```python
from build123d import *

# Parameters (mm, degrees)
F0_R     = 15
F1_DEPTH = 2.5
F2_R     = 5.5
F3_DEPTH = 5
F4_R     = 3
F5_DEPTH = 25
F6_SIZE  = 1


with BuildPart() as f1:
    # F0 (on Front) → F1 (new body)
    with BuildSketch(Plane.XZ):
        Circle(F0_R)
    extrude(amount=F1_DEPTH)

    # F2 (on face) → F3 (join)
    with BuildSketch(Plane.XZ.offset(2.5)):
        Circle(F2_R)
    extrude(amount=F3_DEPTH)

    # F4 (on face) → F5 (cut)
    with BuildSketch(Plane.XZ.offset(7.5)):
        Circle(F4_R)
    extrude(amount=-F5_DEPTH, mode=Mode.SUBTRACT)

    # F6
    f6_edges = [f1.edges().sort_by_distance(p)[0] for p in [
        (-5.5, -7.5, 0),
        (-15, 0, 0),
    ]]
    chamfer(f6_edges, length=F6_SIZE)


solid = f1.part
```
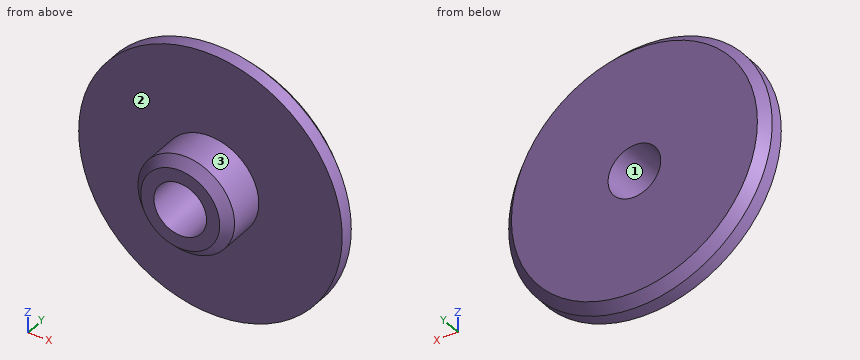
Here's how the part is built. I have some questions about the finished solid (model axes, mm). Face numbers are marked on the shaded views. Give positions to 0.01 mm unless a question says otherwise; leave off trailing zeros. Order: outer loops, then holes, each group sorted by start corner. A loop starts at its lowest first (then second) coordinate and runs counter-clockwise, first axis right, second up. Notation, with made-up numbers: M -3.5,-30 L 40.5,-30 A20 cw 40.5,9 Z; hole C 88,51 d3. An arc over 180 degrees is marked long. Use a Markdown table: item, result. Add a question column.
1. Suppose I cut it at B-B (z = 0). List the corners of the cut face in (x, y) for me, and give its area (3 significant figures).
2. Suppose I cut it at C-C (y = -1.5). List the corners of the cut face in (x, z) for me, and give its area (3 significant figures).
3. Suppose I cut it at A-A (x = 0). List the corners of the cut face in (y, z) for me, and give its area (3 significant figures).
4. Suppose I cut it at D-D (y = -3.5). List the corners of the cut face in (x, z) for me.
5. If we mould it in two halves opening along X, with no side actions, what happens to the marked faces 1, 2 and 3? For each: +X half, -X half, draft (parallel to the pull), parting line (faces both ways), or undercut.
6. I need wall thicknesses on probe 1 along Z at (x, y) = (0, -3.75); probe 2 along Z at (x, y) = (0, -2.25); probe 3 along Y at (x, z) = (-2, -6). Which ranges of each line are inside material? Lowest first, please. Write a range as from..to.
7. For pin 1 Ø3 at (x, z) = (11.5, 10.5) entering from -Y; pin 2 Ø1.5 at (y, z) = (-3, 5.5) entering from +X; pin 3 Ø2 at (y, z) = (-3, 1) entering from -X, each with a flat end and sliding along its axis, tell me the tip position at first contact or that it passes through.
Results list:
| question | item | result |
|---|---|---|
| 1 | outline | M -15,-2.5 L -5.5,-2.5 L -5.5,-6.5 L -4.5,-7.5 L -3,-7.5 L -3,0 L -14,0 L -15,-1 Z; M 3,-7.5 L 4.5,-7.5 L 5.5,-6.5 L 5.5,-2.5 L 15,-2.5 L 15,-1 L 14,0 L 3,0 Z |
| 1 | area | 83.0 mm² |
| 2 | outline | C 0,0 d30; hole C 0,0 d6 |
| 2 | area | 679 mm² |
| 3 | outline | M -7.5,-4.5 L -6.5,-5.5 L -2.5,-5.5 L -2.5,-15 L -1,-15 L 0,-14 L 0,-3 L -7.5,-3 Z; M -7.5,3 L 0,3 L 0,14 L -1,15 L -2.5,15 L -2.5,5.5 L -6.5,5.5 L -7.5,4.5 Z |
| 3 | area | 83.0 mm² |
| 4 | outline | C 0,0 d11; hole C 0,0 d6 |
| 5 | face 1 | undercut |
| 5 | face 2 | draft |
| 5 | face 3 | parting line |
| 6 | probe 1 | z = -5.5..-3, 3..5.5 |
| 6 | probe 2 | z = -15..-3, 3..15 |
| 6 | probe 3 | y = -2.5..0 |
| 7 | pin 1 | stops at y = -2.5 |
| 7 | pin 2 | stops at x = 14.16 |
| 7 | pin 3 | stops at x = -15 |
